Build history of the part. All positions in model axes, mm. A direction names the side the tool comes from. Round coordinates to 2 decimals unless told otherwise and drop trailing zeros. Write each loop counter-clockwise with the first axis right and the second up, starting at its lowest first coordinate (ties: lowest second). Pieces come first, ordered by that corner, then holes. Notation, with made-up numbers: (-19, 54.5) - (18, 54.5) arc R18 cw to (18, 86.5) - close; hole circle Ø11 at (61, -13.5). An arc over 180 degrees is marked (long way). One line per question, with ' | ' between items.
Autodesk Inventor part; units mm, degrees
ref_plane "YZ Plane" through (0, 0, 0) normal (1, 0, 0) x (0, 1, 0)
ref_plane "XZ Plane" through (0, 0, 0) normal (0, 1, 0) x (-1, 0, 0)
ref_plane "XY Plane" through (0, 0, 0) normal (0, 0, 1) x (1, 0, 0)
sketch "Sketch1" plane through (0, 0, 0) normal (0, 0, 1) x (1, 0, 0)
  line L0 (19.685, -19.685) -> (-19.685, -19.685)
  line L1 (-19.685, -19.685) -> (-19.685, 19.685)
  line L2 (-19.685, 19.685) -> (19.685, 19.685)
  line L3 (19.685, 19.685) -> (19.685, -19.685)
  line L4 (19.685, -19.685) -> (-19.685, 19.685) construction
  line L5 (-19.685, -19.685) -> (19.685, 19.685) construction
  line L6 (26.035, 26.035) -> (-26.035, 26.035)
  line L7 (-26.035, 26.035) -> (-26.035, -26.035)
  line L8 (-26.035, -26.035) -> (26.035, -26.035)
  line L9 (26.035, -26.035) -> (26.035, 26.035)
  point P0 (0, 0)
  dimension "d0" = 39.37
  dimension "d1" = 39.37
  dimension "d2" = 6.35
extrude "Extrusion1" add sketch "Sketch1" along normal blind 63.5
sketch "Sketch2" plane through (26.035, -26.035, 0) normal (1, 0, 0) x (0, 0, -1)
  line L0 (-63.5, 45.72) -> (-63.5, 6.35) construction
  line L1 (-63.5, 26.035) -> (50.8, 26.035) construction
  circle A0 centre (12.7, 26.035) radius 7.25
  line L2 (0, 0) -> (0, 52.07)
  circle A1 centre (12.7, 26.035) radius 12.7
  line L3 (0, 52.07) -> (-63.5, 52.07)
  line L4 (0, 52.07) -> (20.5177, 36.0436)
  line L5 (0, 0) -> (-63.5, 0)
  line L6 (0, 0) -> (20.5177, 16.0264)
  point P0 (0, 26.035)
  dimension "d5" = 114.3
  dimension "d6" = 14.5
  dimension "d7" = 12.7
  dimension "d8" = 25.4
extrude "Extrusion2" add sketch "Sketch2" against normal up to surface (52.07 mm away)
sketch "Sketch3" plane through (26.035, -26.035, 63.5) normal (1, 0, 0) x (0, 0, -1)
  circle A0 centre (76.2, 26.035) radius 7.25
  line L0 (63.5, 52.07) -> (0, 52.07)
  line L1 (0, 0) -> (0, 52.07)
  line L2 (63.5, 0) -> (0, 0)
  line L3 (63.5, 0) -> (84.0177, 16.0264)
  arc A1 (84.0177, 16.0264) -> (84.0177, 36.0436) centre (76.2, 26.035) ccw
  line L4 (84.0177, 36.0436) -> (63.5, 52.07)
  line L5 (63.5, 45.72) -> (63.5, 6.35) construction
  circle A2 centre (57.15, 36.83) radius 2.25
  line L6 (63.5, 45.72) -> (0, 45.72) construction
  line L7 (63.5, 45.72) -> (0, 45.72) construction
  line L8 (63.5, 6.35) -> (0, 6.35) construction
  line L9 (63.5, 6.35) -> (0, 6.35) construction
  circle A3 centre (57.15, 15.24) radius 2.25
  circle A4 centre (38.1, 36.83) radius 2.25
  circle A5 centre (38.1, 15.24) radius 2.25
  point P0 (63.5, 26.035)
  dimension "d11" = 4.5
  dimension "d12" = 6.35
  dimension "d13" = 8.89
  dimension "d14" = 4.5
  dimension "d15" = 6.35
  dimension "d16" = 8.89
  dimension "d17" = 4.5
  dimension "d18" = 19.05
  dimension "d19" = 8.89
  dimension "d20" = 4.5
  dimension "d21" = 19.05
  dimension "d22" = 8.89
extrude "Extrusion3" cut sketch "Sketch3" against normal through all contours A2 | A3 | A4 | A5
sketch "Sketch5" plane through (-26.035, 26.035, 0) normal (0, 0.7880827, -0.6155694) x (1, 0, 0)
  line L0 (0, 26.035) -> (0, 0)
  line L1 (52.07, 0) -> (0, 0)
  line L2 (52.07, 26.035) -> (52.07, 0)
  line L3 (52.07, 26.035) -> (0, 26.035)
  line L4 (6.35, 3.9089) -> (45.72, 3.9089) construction
  line L5 (26.035, 3.9089) -> (26.035, 26.035) construction
  line L6 (6.35, 15.4171) -> (0, 15.4171) construction
  line L7 (0, 15.4171) -> (52.07, 15.4171) construction
  line L8 (52.07, 15.4171) -> (45.72, 15.4171) construction
  line L9 (45.085, 19.1671) -> (6.985, 19.1671)
  line L10 (6.985, 19.1671) -> (6.985, 11.6671)
  line L11 (6.985, 11.6671) -> (45.085, 11.6671)
  line L12 (45.085, 11.6671) -> (45.085, 19.1671)
  line L13 (45.085, 19.1671) -> (6.985, 11.6671) construction
  line L14 (6.985, 19.1671) -> (45.085, 11.6671) construction
  point P0 (26.035, 16.0264)
  point P1 (26.035, 15.4171)
  dimension "d30" = 38.1
  dimension "d31" = 7.5
extrude "Extrusion5" cut sketch "Sketch5" against normal up to surface contours L12 L11 L10 L9 surface through (19.685, -19.685, 0) normal (0, 1, 0)
properties part number "CS_Climb_Outer_Tube_End_Cap"
Q1. Saw through at B-B, the plane z = 25.4. List the corners of the cut face in (x, y) (3 decimals), then the cut area to 3 significant figures.
Found:
outline: (-26.035, -26.035) - (26.035, -26.035) - (26.035, -13.045) - (19.685, -13.045) - (19.685, -19.685) - (-19.685, -19.685) - (-19.685, -13.045) - (-26.035, -13.045) - close; (-26.035, -8.545) - (-19.685, -8.545) - (-19.685, 8.545) - (-26.035, 8.545) - close; (-26.035, 13.045) - (-19.685, 13.045) - (-19.685, 19.685) - (19.685, 19.685) - (19.685, 13.045) - (26.035, 13.045) - (26.035, 26.035) - (-26.035, 26.035) - close; (19.685, -8.545) - (26.035, -8.545) - (26.035, 8.545) - (19.685, 8.545) - close | area: 1,050 mm^2
Q2. Saw through at A-A, the plane z = 51. List the corners of the cut face in (x, y) (3 decimals).
Found:
outline: (-26.035, -26.035) - (26.035, -26.035) - (26.035, 26.035) - (-26.035, 26.035) - close; hole (-19.685, -19.685) - (19.685, -19.685) - (19.685, 19.685) - (-19.685, 19.685) - close
Q3. Which spindle directions (+Z, -Z, +X, -X, +Y, -Y) get a long thin tool onto all of the face, cutting with end or side? Do faces 4 (the cylindrical face through (22.9, 12.7, 24.2)), 5 (the flat face through (-19.685, 0, 31)), 6 (the flat face through (19.05, 9, -6)). Say none if no direction does.
Found:
face 4: +X, -X | face 5: +Z | face 6: none
Q4. Drop flat-ended pins along their axis: pin 1 (2 mm diameter, centred on x = 14, y = 19.5, fed in from -Z); pin 2 (4 mm diameter, centred on y = 10.795, z = 6.35, fed in from -X); pin 3 (5 mm diameter, centred on x = 8, y = 16.5, fed in from +Z); pin 4 (4 mm diameter, centred on x = -13, y = -17.5, fed in from -Z). Give the stop position or say it passes through.
Found:
pin 1: z = -9.19 | pin 2: through | pin 3: z = 0 | pin 4: z = -13.49
Q5. Drill centre lines: L1, parallel to Y at x = 22.5, z = 25.4 (3 decimals); L2, parallel to Y at x = 9, z = 49 (3 decimals); L3, parallel to Z at x = 24.5, y = 11. Where is each one in solid material? Low to high. Write a range as from..to.
Found:
L1: -26.035..-13.045, -8.545..8.545, 13.045..26.035 | L2: -26.035..-19.685, 19.685..26.035 | L3: -19.25..4.11, 8.59..23.16, 27.64..63.5
Q6. Saw through at C-C, the plane x = 0.5. List the corners of the cut face in (y, z) (3 decimals), then the cut area to 3 significant figures.
Found:
outline: (-26.035, 0) - (-10.009, -20.518) arc R12.7 ccw to (10.009, -20.518) - (14.236, -15.105) - (6.058, -8.717) arc R7.25 cw (long way) to (2.397, -5.858) - (-5.102, 0) - (-19.685, 0) - (-19.685, 63.5) - (-26.035, 63.5) - close; (7.082, 0) - (18.853, -9.195) - (26.035, 0) - (26.035, 63.5) - (19.685, 63.5) - (19.685, 0) - close | area: 1,300 mm^2
Q7. Saw through at D-D, the plane y = 0. List the corners of the cut face in (x, z) (3 decimals).
Found:
outline: (-26.035, -25.4) - (26.035, -25.4) - (26.035, -19.95) - (-26.035, -19.95) - close; (-26.035, -5.45) - (26.035, -5.45) - (26.035, 63.5) - (19.685, 63.5) - (19.685, 0) - (19.05, 0) - (19.05, -3.985) - (-19.05, -3.985) - (-19.05, 0) - (-19.685, 0) - (-19.685, 63.5) - (-26.035, 63.5) - close
Q8. Pull direction X, two halves, no side cores. Call faces 1 (the flat face through (0.36, -18.13, -10.12)), 2 (the flat face through (-26.035, 0, 28)), 3 (the flat face through (19.685, 0, 31)): +X half, -X half, draft (parallel to the pull), parting line (faces both ways), or undercut.
Found:
face 1: draft | face 2: -X half | face 3: undercut
